The drawing under review shows one solid part. Ordinate dimensions are in mm from its lowest x, y, z. A direction names the side the tool comes from. Give positions to 0.01 mm unless a question says otherwise; leave off trailing zeros. Order: outer loops, then holes, each group sorted by start corner. A loop starts at its lowest first (then second) coordinate and runs counter-clockwise, first axis right, second up. Notation, with made-up numbers: (28, 56.5) -> (75, 56.5) arc R29 ccw to (75, 80.5) -> close; hole circle Ø8 at (79.5, -23.5). An arc over 180 degrees is marked (long way). Use a Markdown table: item, result. Add a question column.
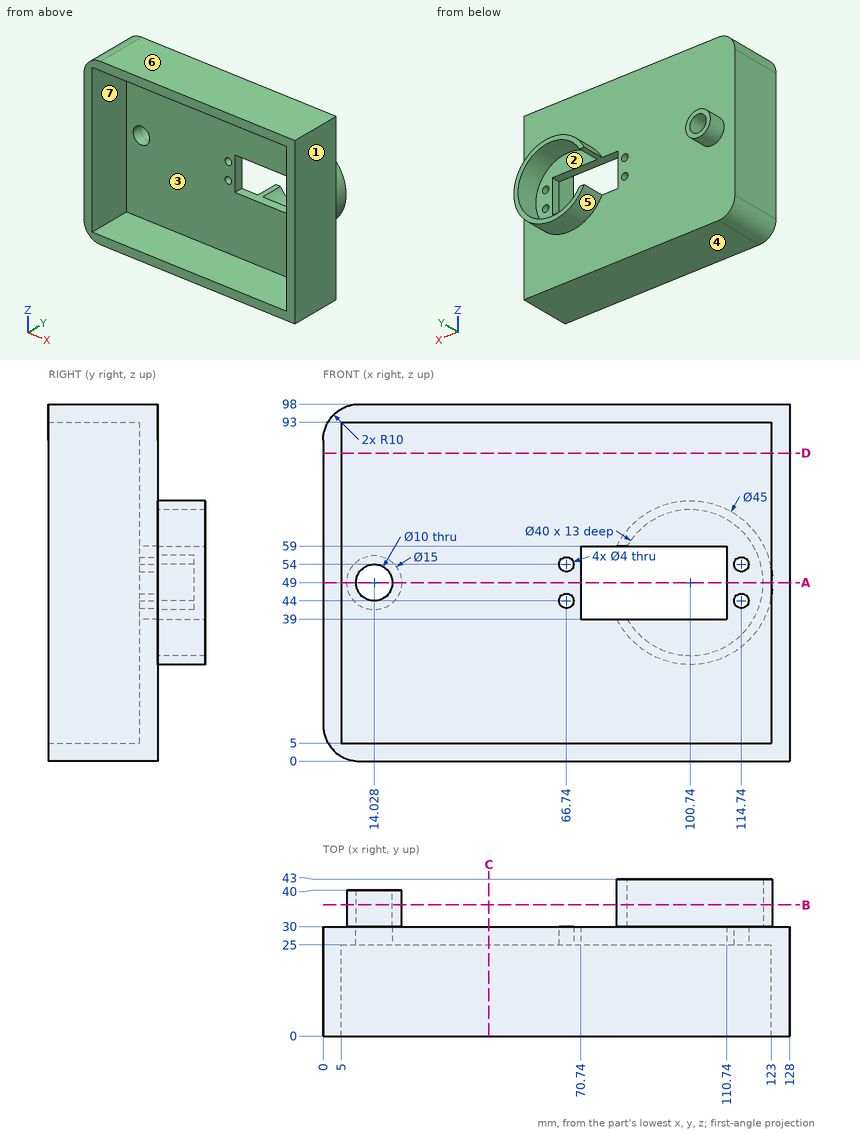
1) Insertion check: pin 1 (8 mm diameter, centred on x = 110.5, z = 85.5, fed in from -Y); pin 2 (9 mm diameter, centred on x = 14.03, z = 49, fed in from -Y); pin 3 (1 mm diameter, centred on x = 73.5, z = 20.5, fed in from +Y); pin 4 (2 mm diameter, centred on x = 21, y = 38, fed in from +Z). Each pin has a flat end and moves straight along its axis. Give the tip position at first contact, or say it passes through.
2) Machinability: for the marked faces 1, 2 and 3, which of the approach directions +Z, -Z, +X, -X, +Y, -Y give a long, thin tool a straight path to every point of the face, cutting with its end or side? Answer none if there is none.
3) For L1, parallel to Z at x = 65, y = 13.5; L2, parallel to X at y = 8.5, z = 34; L3, parallel to Z at x = 94, y = 29, list the stretches that pass through material, from the lowest coordinate up. Write a range as [from, to].
4) Add section A-A (z = 49). Give the boundary of the cut face in (x, y).
5) Add section D-D (z = 84.5). Give the boundary of the cut face in (x, y).
6) The part is to be moulded in two halves that separate along Z. For the marked faces 4, 5, 6 and 7, say which applies: +Z half, -Z half, draft (parallel to the pull), parting line (faces both ways), or undercut.
7) Add section B-B (y = 36). Give the boundary of the cut face in (x, z), then the cut area to 3 significant figures.
8) Add section C-C (x = 45.5). Give the boundary of the cut face in (y, z).
Worked answers:
| question | item | result |
|---|---|---|
| 1 | pin 1 | y = 25 |
| 1 | pin 2 | through |
| 1 | pin 3 | y = 30 |
| 1 | pin 4 | z = 53.54 |
| 2 | face 1 | +Z, -Z, +X, +Y, -Y |
| 2 | face 2 | +Y |
| 2 | face 3 | -Y |
| 3 | L1 | [0, 5], [93, 98] |
| 3 | L2 | [0, 5], [123, 128] |
| 3 | L3 | [0, 39], [59, 98] |
| 4 | outline | (0, 0) -> (5, 0) -> (5, 25) -> (9.03, 25) -> (9.03, 40) -> (6.53, 40) -> (6.53, 30) -> (0, 30) -> close; (19.03, 25) -> (70.74, 25) -> (70.74, 30) -> (21.53, 30) -> (21.53, 40) -> (19.03, 40) -> close; (110.74, 25) -> (123, 25) -> (123, 0) -> (128, 0) -> (128, 30) -> (123.24, 30) -> (123.24, 43) -> (120.74, 43) -> (120.74, 30) -> (110.74, 30) -> close |
| 5 | outline | (0, 0) -> (5, 0) -> (5, 25) -> (123, 25) -> (123, 0) -> (128, 0) -> (128, 30) -> (0, 30) -> close |
| 6 | face 4 | -Z half |
| 6 | face 5 | parting line |
| 6 | face 6 | +Z half |
| 6 | face 7 | undercut |
| 7 | outline | circle Ø15 at (14.03, 49); (80.58, 39) arc R22.5 ccw (long way) to (80.58, 59) -> (83.42, 59) arc R20 cw (long way) to (83.42, 39) -> close; hole circle Ø10 at (14.03, 49) |
| 7 | area | 380 mm^2 |
| 8 | outline | (0, 0) -> (30, 0) -> (30, 98) -> (0, 98) -> (0, 93) -> (25, 93) -> (25, 5) -> (0, 5) -> close |
